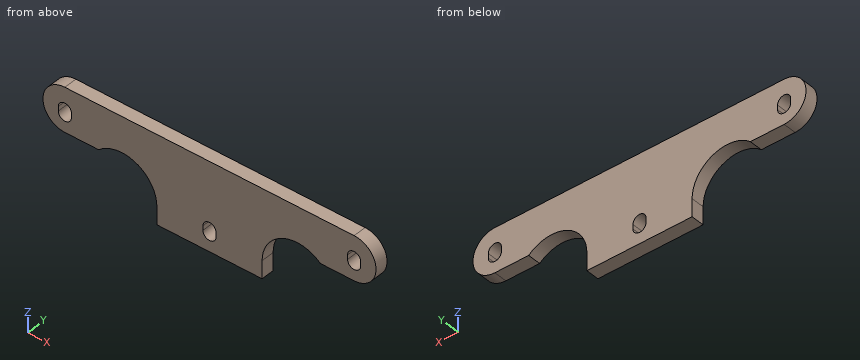
from build123d import *

# Parameters (mm, degrees)
BOSS_EXTRUDE1_DEPTH = 3
CUT_EXTRUDE1_DEPTH  = 44.0464865


with BuildPart() as part:
    # Sketch1 → Boss-Extrude1 (new body)
    with BuildSketch(Plane(origin=(0, 0, 0), x_dir=(1, 0, 0), z_dir=(0, 1, 0))):
        with BuildLine():
            Line((0, 0), (-33, 0))
            ThreePointArc((-33, 0), (-38, 5), (-33, 10))
            Line((-33, 10), (-25.291502622, 10))
            ThreePointArc((-25.291502622, 10), (-16.708497378, 8.708497378), (-12, 16))
            Line((-12, 16), (-12, 20))
            Line((-12, 20), (12, 20))
            Line((12, 20), (12, 16))
            ThreePointArc((12, 16), (16.708497378, 8.708497378), (25.291502622, 10))
            Line((25.291502622, 10), (33, 10))
            ThreePointArc((33, 10), (38, 5), (33, 0))
            Line((33, 0), (0, 0))
        make_face()
    extrude(amount=BOSS_EXTRUDE1_DEPTH)

    # Sketch2 → Cut-Extrude1 (cut, through all)
    with BuildSketch(Plane(origin=(0, 3, 0), x_dir=(1, 0, 0), z_dir=(0, 1, 0))):
        with BuildLine():
            Line((-34.5, 5), (-34.5, 6))
            ThreePointArc((-34.5, 6), (-33, 7.5), (-31.5, 6))
            Line((-31.5, 6), (-31.5, 5))
            ThreePointArc((-31.5, 5), (-33, 3.5), (-34.5, 5))
        make_face()
        with BuildLine():
            Line((31.5, 5), (31.5, 6))
            ThreePointArc((31.5, 6), (33, 7.5), (34.5, 6))
            Line((34.5, 6), (34.5, 5))
            ThreePointArc((34.5, 5), (33, 3.5), (31.5, 5))
        make_face()
        with BuildLine():
            Line((-1.5, 15), (-1.5, 16))
            ThreePointArc((-1.5, 16), (0, 17.5), (1.5, 16))
            Line((1.5, 16), (1.5, 15))
            ThreePointArc((1.5, 15), (0, 13.5), (-1.5, 15))
        make_face()
    extrude(amount=-CUT_EXTRUDE1_DEPTH, mode=Mode.SUBTRACT)


solid = part.part
Input: part model. Units: mm. Frame: model coordinates. Round coordinates to 2 decimals unless told otherwise and drop trailing zeros. Order: outer loops, then holes, each group sorted by start corner. A loop starts at its lowest first (then second) coordinate and runs counter-clockwise, first axis right, second up.
1. Cut plane A-A, the plane x = 0. Output: boundary loops of the cut face in (y, z).
The answers:
outline: (0, -20) - (3, -20) - (3, -17.5) - (0, -17.5) - close; (0, -13.5) - (3, -13.5) - (3, 0) - (0, 0) - close
2. Cut plane D-D, the plane z = -12. Output: boundary loops of the cut face in (x, y), then the cut area to 3 significant figures.
The answers:
outline: (-13.07, 0) - (13.07, 0) - (13.07, 3) - (-13.07, 3) - close
area: 78.4 mm2
3. Pin query (flat end, axial travel): P1, Ø0.9, axis at x = 30, y = 1, coming from the -Z side; P2, Ø0.9, axis at y = 1, z = -18, coming from the +X side. Return the tip coordinate at first contact, or that it passes through.
The answers:
P1: stops at z = -10
P2: stops at x = 12
4. Cut plane C-C, the plane x = 27. Output: boundary loops of the cut face in (y, z), then the cut area to 3 significant figures.
The answers:
outline: (0, -10) - (3, -10) - (3, 0) - (0, 0) - close
area: 30.0 mm2
5. Material intervals for line 1 (X direction, y = 1.15, z = -5); line 2 (X direction, y = 0.6, z = -6.25); line 3 (X direction, y = 0.25, z = -16.5), sorted ascending.
The answers:
line 1: x = -38 to -34.5, -31.5 to 31.5, 34.5 to 38
line 2: x = -37.84 to -34.48, -31.52 to 31.52, 34.48 to 37.84
line 3: x = -12 to -1.41, 1.41 to 12
6. Cut plane B-B, the plane y = 1.2. Output: boundary loops of the cut face in (x, z).
The answers:
outline: (-33, -10) - (-25.29, -10) arc R8 cw to (-12, -16) - (-12, -20) - (12, -20) - (12, -16) arc R8 cw to (25.29, -10) - (33, -10) arc R5 ccw to (33, 0) - (-33, 0) arc R5 ccw to start; hole (-34.5, -6) arc R1.5 ccw to (-31.5, -6) - (-31.5, -5) arc R1.5 ccw to (-34.5, -5) - close; hole (-1.5, -16) arc R1.5 ccw to (1.5, -16) - (1.5, -15) arc R1.5 ccw to (-1.5, -15) - close; hole (31.5, -6) arc R1.5 ccw to (34.5, -6) - (34.5, -5) arc R1.5 ccw to (31.5, -5) - close
